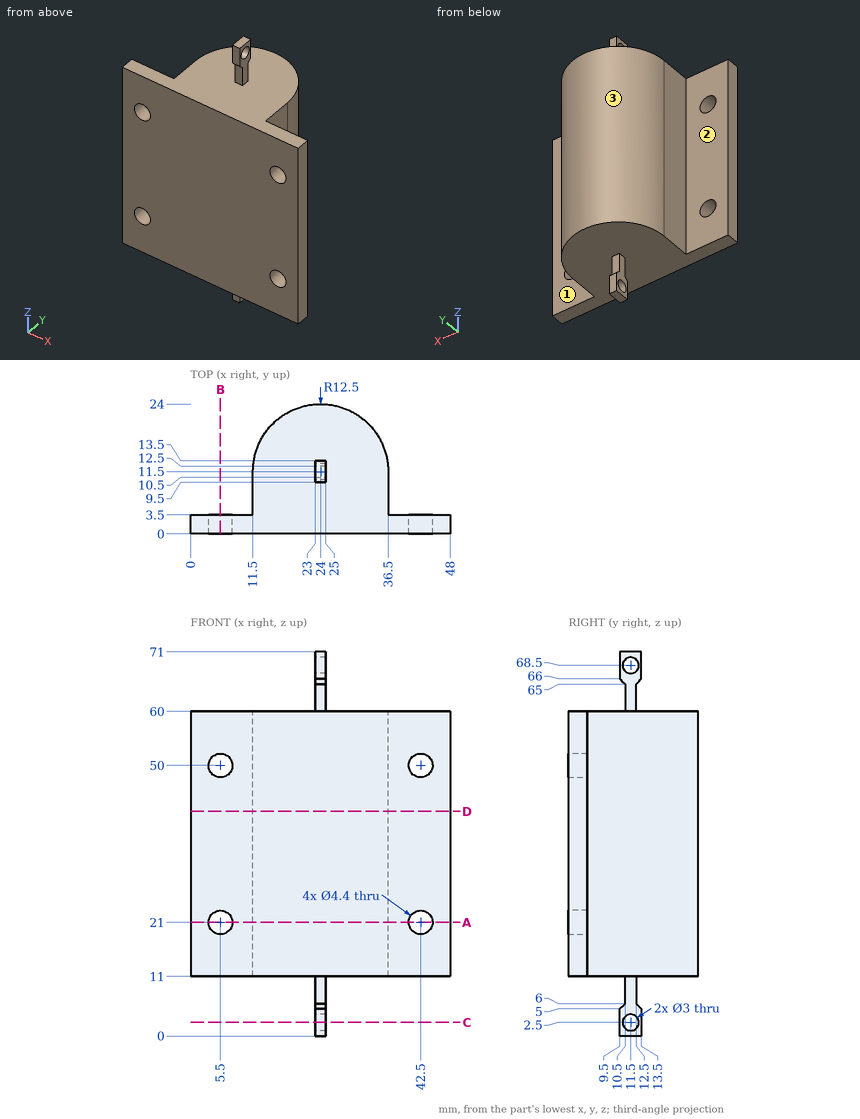
Check sheet for the drawn part. Datum: minimum x, y, z corner. Units: mm. A direction names the side the tool comes from. Coordinates: 2 decimals unless noted, no trailing zeros. Write each loop counter-clockwise with the first axis right and the second up, starting at its lowest first coordinate (ties: lowest second). Pieces come first, ordered by that corner, then holes. Notation, with made-up numbers: M -27,51.25 L -7,51.25 A19 cw -7,67.25 Z; hole C -33.5,-30 d3. An arc over 180 degrees is marked long. One line per item, written item: value.
Item 1: Section check C-C, the plane z = 2.5. Record the boundary of the cut face in (x, y).
Check sheet entries:
outline: M 23,9.5 L 25,9.5 L 25,10 L 23,10 Z; M 23,13 L 25,13 L 25,13.5 L 23,13.5 Z
Item 2: Section check A-A, the plane z = 21. Record the boundary of the cut face in (x, y), plus the area to 3 significant figures.
Check sheet entries:
outline: M 0,0 L 3.3,0 L 3.3,3.5 L 0,3.5 Z; M 7.7,0 L 40.3,0 L 40.3,3.5 L 36.5,3.5 L 36.5,11.5 A12.5 ccw 11.5,11.5 L 11.5,3.5 L 7.7,3.5 Z; M 44.7,0 L 48,0 L 48,3.5 L 44.7,3.5 Z
area: 583 mm^2
Item 3: Scan lines: line 1 along X through (y, z) = (1.4, 21); line 2 along Y through (x, z) = (40, 25); line 3 along Z through (x, y) = (4.5, 2). Record each from-to range of solid material in increasing order.
Check sheet entries:
line 1: x = 0 to 3.3, 7.7 to 40.3, 44.7 to 48
line 2: y = 0 to 3.5
line 3: z = 11 to 19.04, 22.96 to 48.04, 51.96 to 60
Item 4: Section check D-D, the plane z = 41.5. Record the boundary of the cut face in (x, y), plus the area to 3 significant figures.
Check sheet entries:
outline: M 0,0 L 48,0 L 48,3.5 L 36.5,3.5 L 36.5,11.5 A12.5 ccw 11.5,11.5 L 11.5,3.5 L 0,3.5 Z
area: 613 mm^2
Item 5: Gauge pin test, flat ends, axial feed: pin 1 Ø1 at (x, y) = (27, 8.5) entering from -Z; pin 2 Ø6 at (x, z) = (42, 38.5) entering from +Y; pin 3 Ø2.5 at (y, z) = (11.5, 2.5) entering from -X; pin 4 Ø2 at (x, y) = (19, 19) entering from +Z. Record the tip position at first contact, or that the pin passes through.
Check sheet entries:
pin 1: stops at z = 11
pin 2: stops at y = 3.5
pin 3: passes through
pin 4: stops at z = 60
Item 6: Section check B-B, the plane x = 5.5. Record the boundary of the cut face in (y, z).
Check sheet entries:
outline: M 0,11 L 3.5,11 L 3.5,18.8 L 0,18.8 Z; M 0,23.2 L 3.5,23.2 L 3.5,47.8 L 0,47.8 Z; M 0,52.2 L 3.5,52.2 L 3.5,60 L 0,60 Z
Item 7: Access from +Z, -Z, +X, -X, +Y, -Y to the whole of each face (thin tool, end or side, straight path). Record for the marked faces 1, 2 and 3.
Check sheet entries:
face 1: +Z, -Z, +X, +Y
face 2: +Z, -Z, -X, +Y
face 3: +Z, -Z, +Y
